Check sheet for the drawn part. Datum: minimum x, y, z corner. Units: mm. Give positions to 0.01 mm unless a question says otherwise; leave off trailing zeros. Loops run counter-clockwise (first coordinate to the right, second up) from the corner with the lowest first, then second, coordinate; pieces in that order, holes last.
1. Cross-section at A-A, the plane x = 138.5. Record the cut outline in (y, z).
2. Cross-section at B-B, the plane z = 32.5. Record the cut outline in (x, y), plus the area to 3 significant figures.
3. Go/stop test with a flat-tipped pin: pin 1 Ø3 at (y, z) = (8.5, 45) entering from -X. Record where the tip stops, or that it passes through.
4. Cross-section at C-C, the plane y = 8. Record the cut outline in (x, z).
5. Cross-section at D-D, the plane x = 64.5. Record the cut outline in (y, z), plus the area to 3 significant figures.
6. Material ranges on L1, parallel to X at y = 2, z = 32.5; L2, parallel to Z at x = 138.5, y = 3.75; L3, parallel to X at y = 4.25, z = 32.5, recorded low to high.
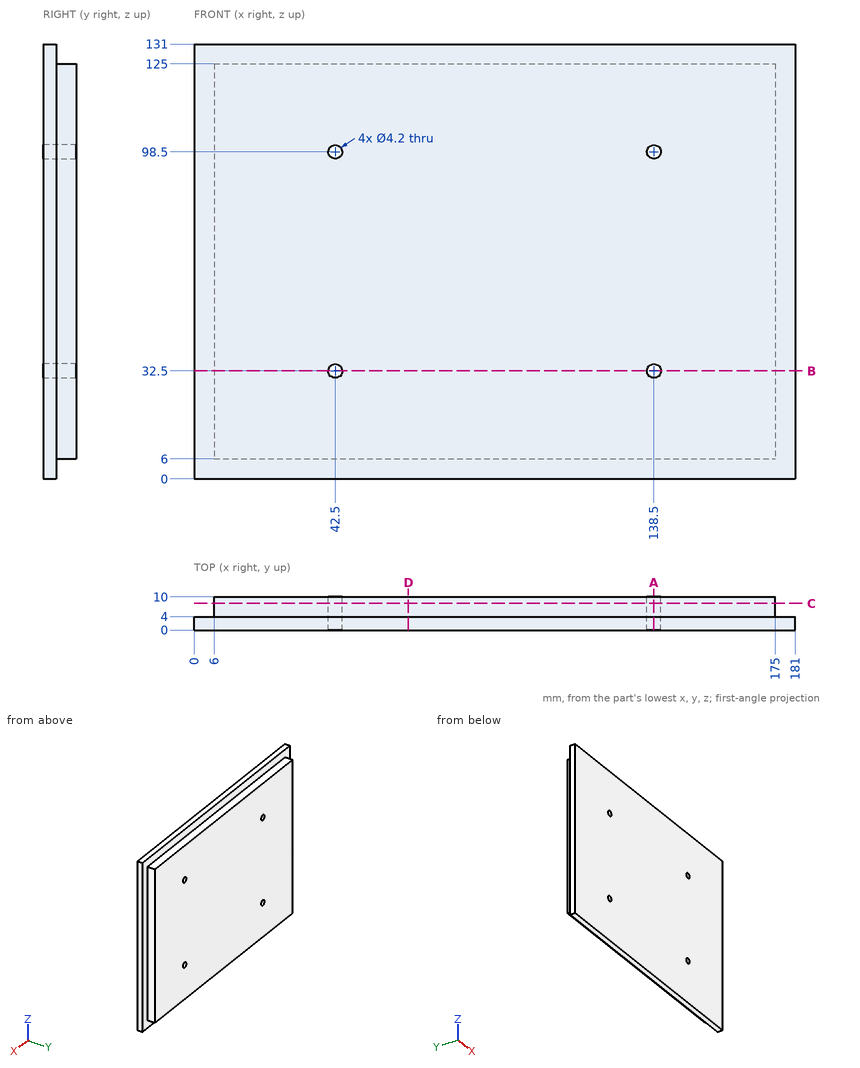
Result:
1. outline: (0, 0) - (4, 0) - (4, 6) - (10, 6) - (10, 30.4) - (0, 30.4) - close; (0, 34.6) - (10, 34.6) - (10, 96.4) - (0, 96.4) - close; (0, 100.6) - (10, 100.6) - (10, 125) - (4, 125) - (4, 131) - (0, 131) - close
2. outline: (0, 0) - (40.4, 0) - (40.4, 10) - (6, 10) - (6, 4) - (0, 4) - close; (44.6, 0) - (136.4, 0) - (136.4, 10) - (44.6, 10) - close; (140.6, 0) - (181, 0) - (181, 4) - (175, 4) - (175, 10) - (140.6, 10) - close
2. area: 1,650 mm2
3. pin 1: stops at x = 6
4. outline: (6, 6) - (175, 6) - (175, 125) - (6, 125) - close; hole circle Ø4.2 at (42.5, 32.5); hole circle Ø4.2 at (42.5, 98.5); hole circle Ø4.2 at (138.5, 32.5); hole circle Ø4.2 at (138.5, 98.5)
5. outline: (0, 0) - (4, 0) - (4, 6) - (10, 6) - (10, 125) - (4, 125) - (4, 131) - (0, 131) - close
5. area: 1,240 mm2
6. L1: x = 0 to 40.4, 44.6 to 136.4, 140.6 to 181
6. L2: z = 0 to 30.4, 34.6 to 96.4, 100.6 to 131
6. L3: x = 6 to 40.4, 44.6 to 136.4, 140.6 to 175
